from build123d import *

# Parameters (mm, degrees)
SKETCH1_R               = 4.70408
BOSS_EXTRUDE1_DEPTH     = 58.02376
CUT_EXTRUDE1_DEPTH      = 5.70408
CUT_EXTRUDE1_DEPTH_BACK = 5.70408
SKETCH3_R               = 6.2738
CUT_EXTRUDE2_DEPTH      = 5.704080123
SKETCH4_R               = 1.56718
CUT_EXTRUDE3_DEPTH      = 5.7040801


with BuildPart() as part:
    # Sketch1 → Boss-Extrude1 (new body)
    with BuildSketch(Plane(origin=(0, 0, 0), x_dir=(0, 0, -1), z_dir=(1, 0, 0))):
        Circle(SKETCH1_R)
    extrude(amount=-BOSS_EXTRUDE1_DEPTH)

    # Sketch2 → Cut-Extrude1 (cut, two sides)
    with BuildSketch(Plane.XY) as cut_extrude1_sk:
        with BuildLine():
            Line((-6.2738, 6.2738), (2.931020603, 6.2738))
            Line((2.931020603, 6.2738), (2.931020603, -6.2738))
            Line((2.931020603, -6.2738), (-6.2738, -6.2738))
            ThreePointArc((-6.2738, -6.2738), (0, 0), (-6.2738, 6.2738))
        make_face()
    extrude(amount=CUT_EXTRUDE1_DEPTH, mode=Mode.SUBTRACT)
    extrude(cut_extrude1_sk.sketch, amount=-CUT_EXTRUDE1_DEPTH_BACK, mode=Mode.SUBTRACT)

    # Sketch3 → Cut-Extrude2 (cut, through all)
    with BuildSketch(Plane.XY):
        with Locations((-4.70408, 0)):
            Circle(SKETCH3_R)
    extrude(amount=CUT_EXTRUDE2_DEPTH, mode=Mode.SUBTRACT)

    # Sketch4 → Cut-Extrude3 (cut, through all)
    with BuildSketch(Plane.XY):
        with Locations((-5.09524, 0)):
            Circle(SKETCH4_R)
    extrude(amount=-CUT_EXTRUDE3_DEPTH, mode=Mode.SUBTRACT)


solid = part.part
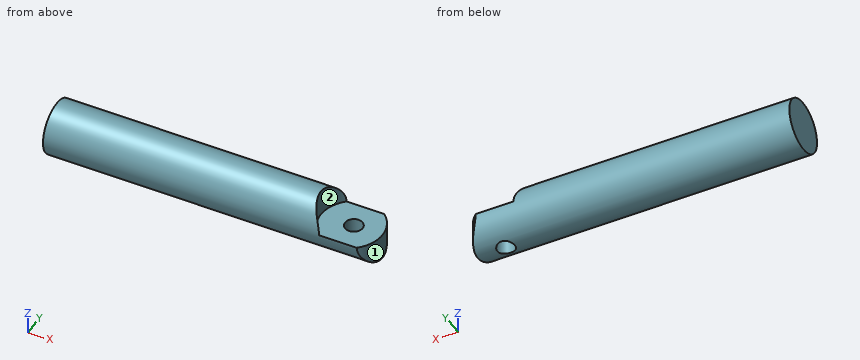
Check sheet for the modelled part. Datum: model origin and axes. Units: mm. Face numbers are marked on the shaded views. A direction names the side the tool comes from. Round coordinates to 2 decimals unless told otherwise and drop trailing zeros. Loops run counter-clockwise (first coordinate to the right, second up) from the corner with the lowest first, then second, coordinate; pieces in that order, holes last. Notation, with made-up numbers: M 54.5,-0.75 L 113.5,-0.75 A35 ccw 113.5,38.25 Z; hole C 29,-38 d8. An arc over 180 degrees is marked long. One line per question, with ' | ' between items. Start each with the question number.
Item 1: Section check A-A (y = 0). Record the boundary of the cut face in (x, z), and give its area (3 significant figures).
Item 2: Section check D-D (y = 4). Record the boundary of the cut face in (x, z), and give its area (3 significant figures).
Item 3: Gauge pin test, flat ends, axial feed: pin 1 Ø1.5 at (x, y) = (-22, 1) entering from +Z; pin 2 Ø4.5 at (x, y) = (-6.5, 1.5) entering from +Z; pin 3 Ø2 at (x, z) = (-23, 3) entering from +Y. Record the tip position at first contact, or that the pin passes through.
Item 4: Section check B-B (z = -4). Record the boundary of the cut face in (x, y).
Item 5: Set-up check for the marked faces 1 and 2: record each of +Z, -Z, +X, -X, +Y, -Y from which the full face is reachable in a straight line by a thin tool's end or side.
Item 6: Scan lines: probe 1 along X at (y, z) = (0, -1.15); probe 2 along Z at (x, y) = (-8.5, 0.25); probe 3 along Y at (x, z) = (-31.5, 2.75). Record each from-to range of solid material in increasing order.
Item 7: Section check C-C (x = -30). Record the boundary of the cut face in (y, z).
Worked out:
1) outline: M -58.02,-4.7 L -6.66,-4.7 L -6.66,0 L -10.98,0 L -10.98,4.7 L -58.02,4.7 Z; M -3.53,-4.7 L 0,-4.7 L 0,0 L -3.53,0 Z | area: 480 mm^2
2) outline: M -58.02,-2.48 L -1.44,-2.48 L -1.44,0 L -9.54,0 L -9.54,2.48 L -58.02,2.48 Z | area: 260 mm^2
3) pin 1: z = 4.7 | pin 2: z = 0 | pin 3: y = 4.26
4) outline: M -58.02,-2.48 L -0.51,-2.48 A6.27 ccw -0.51,2.48 L -58.02,2.48 Z; hole C -5.1,0 d3.13
5) face 1: +Z, -Z, +X | face 2: +Z, +X
6) probe 1: -58.02 to -6.66, -3.53 to 0 | probe 2: -4.7 to 0 | probe 3: -3.82 to 3.82
7) outline: C 0,0 d9.41
